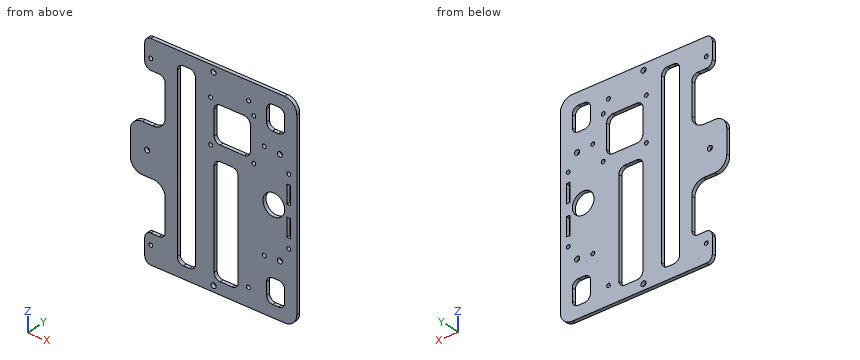
```python
from build123d import *

# Parameters (mm, degrees)
SKETCH1_W           = 138
SKETCH1_H           = 170
BOSS_EXTRUDE1_DEPTH = 3
SKETCH2_R           = 2.1
SKETCH2_W           = 29
SKETCH2_H           = 30
CUT_EXTRUDE1_DEPTH  = 3
SKETCH3_R           = 2.1
CUT_EXTRUDE2_DEPTH  = 219.981734398
SKETCH5_W           = 29
SKETCH5_H           = 35
CUT_EXTRUDE3_DEPTH  = 219.981734398
SKETCH6_R           = 1.6
SKETCH6_W           = 3.2
SKETCH6_H           = 15.2
CUT_EXTRUDE4_DEPTH  = 219.981734398
SKETCH9_W           = 29
SKETCH9_H           = 30
BOSS_EXTRUDE2_DEPTH = 3
SKETCH10_R          = 1.6
CUT_EXTRUDE5_DEPTH  = 219.981734398
FILLET1_R           = 10
FILLET2_R           = 10
SKETCH12_W          = 15
SKETCH12_H          = 150
CUT_EXTRUDE6_DEPTH  = 219.981734398
FILLET3_R           = 5
SKETCH13_R          = 9
SKETCH13_W          = 15
SKETCH13_H          = 20
CUT_EXTRUDE7_DEPTH  = 219.981734398
FILLET4_R           = 5
SKETCH14_W          = 27
SKETCH14_H          = 24
SKETCH14_R          = 1.6
BOSS_EXTRUDE3_DEPTH = 3
SKETCH15_R          = 1.6
CUT_EXTRUDE8_DEPTH  = 219.981734398
FILLET5_R           = 5
SKETCH16_W          = 20
SKETCH16_H          = 90
CUT_EXTRUDE9_DEPTH  = 219.981734398
FILLET6_R           = 5


with BuildPart() as part:
    # Sketch1 → Boss-Extrude1 (new body)
    with BuildSketch(Plane(origin=(0, 0, 0), x_dir=(1, 0, 0), z_dir=(0, 1, 0))):
        with Locations((69, 85)):
            Rectangle(SKETCH1_W, SKETCH1_H)
    extrude(amount=BOSS_EXTRUDE1_DEPTH)

    # Sketch2 → Cut-Extrude1 (cut)
    with BuildSketch(Plane(origin=(0, 3, 0), x_dir=(1, 0, 0), z_dir=(0, 1, 0))):
        with Locations(Location((69, 165, 0), (0, 0, 270))):
            Circle(SKETCH2_R)
        with Locations(Location((69, 5, 0), (0, 0, 270))):
            Circle(SKETCH2_R)
        with Locations((14.5, 155)):
            Rectangle(SKETCH2_W, SKETCH2_H)
        with Locations((123.5, 155)):
            Rectangle(SKETCH2_W, SKETCH2_H)
        with Locations((123.5, 15)):
            Rectangle(SKETCH2_W, SKETCH2_H)
        with Locations((14.5, 15)):
            Rectangle(SKETCH2_W, SKETCH2_H)
    extrude(amount=-CUT_EXTRUDE1_DEPTH, mode=Mode.SUBTRACT)

    # Sketch3 → Cut-Extrude2 (cut, through all)
    with BuildSketch(Plane(origin=(0, 3, 0), x_dir=(1, 0, 0), z_dir=(0, 1, 0))):
        with Locations(Location((14, 125, 0), (0, 0, 270))):
            Circle(SKETCH3_R)
        with Locations(Location((14, 45, 0), (0, 0, 270))):
            Circle(SKETCH3_R)
        with Locations(Location((14, 85, 0), (0, 0, 270))):
            Circle(SKETCH3_R)
        with Locations(Location((124, 45, 0), (0, 0, 90))):
            Circle(SKETCH3_R)
        with Locations(Location((124, 125, 0), (0, 0, 90))):
            Circle(SKETCH3_R)
    extrude(amount=-CUT_EXTRUDE2_DEPTH, mode=Mode.SUBTRACT)

    # Sketch5 → Cut-Extrude3 (cut, through all)
    with BuildSketch(Plane(origin=(0, 3, 0), x_dir=(1, 0, 0), z_dir=(0, 1, 0))):
        with Locations((14.5, 122.5)):
            Rectangle(SKETCH5_W, SKETCH5_H)
        with Locations((14.5, 47.5)):
            Rectangle(SKETCH5_W, SKETCH5_H)
    extrude(amount=-CUT_EXTRUDE3_DEPTH, mode=Mode.SUBTRACT)

    # Sketch6 → Cut-Extrude4 (cut, through all)
    with BuildSketch(Plane(origin=(0, 3, 0), x_dir=(1, 0, 0), z_dir=(0, 1, 0))):
        with Locations(Location((131.4, 113, 0), (0, 0, 270))):
            Circle(SKETCH6_R)
        with Locations(Location((131.4, 57, 0), (0, 0, 270))):
            Circle(SKETCH6_R)
        with Locations((131.4, 97.4)):
            Rectangle(SKETCH6_W, SKETCH6_H)
        with Locations((131.4, 72.6)):
            Rectangle(SKETCH6_W, SKETCH6_H)
    extrude(amount=-CUT_EXTRUDE4_DEPTH, mode=Mode.SUBTRACT)

    # Sketch9 → Boss-Extrude2 (add)
    with BuildSketch(Plane(origin=(0, 3, 0), x_dir=(1, 0, 0), z_dir=(0, 1, 0))):
        with Locations((123.5, 155)):
            Rectangle(SKETCH9_W, SKETCH9_H)
        with Locations((123.5, 15)):
            Rectangle(SKETCH9_W, SKETCH9_H)
    extrude(amount=-BOSS_EXTRUDE2_DEPTH)

    # Sketch10 → Cut-Extrude5 (cut, through all)
    with BuildSketch(Plane(origin=(0, 3, 0), x_dir=(1, 0, 0), z_dir=(0, 1, 0))):
        with Locations(Location((66.6, 60.4, 0), (0, 0, 270))):
            Circle(SKETCH10_R)
        with Locations(Location((102.4, 60.4, 0), (0, 0, 270))):
            Circle(SKETCH10_R)
        with Locations(Location((66.6, 24.6, 0), (0, 0, 270))):
            Circle(SKETCH10_R)
        with Locations(Location((102.4, 24.6, 0), (0, 0, 270))):
            Circle(SKETCH10_R)
        with BuildLine():
            Line((74.5, 57.5), (94.5, 57.5))
            ThreePointArc((94.5, 57.5), (98.035533906, 56.035533906), (99.5, 52.5))
            Line((99.5, 52.5), (99.5, 32.5))
            ThreePointArc((99.5, 32.5), (98.035533906, 28.964466094), (94.5, 27.5))
            Line((94.5, 27.5), (74.5, 27.5))
            ThreePointArc((74.5, 27.5), (70.964466094, 28.964466094), (69.5, 32.5))
            Line((69.5, 32.5), (69.5, 52.5))
            ThreePointArc((69.5, 52.5), (70.964466094, 56.035533906), (74.5, 57.5))
        make_face()
    extrude(amount=-CUT_EXTRUDE5_DEPTH, mode=Mode.SUBTRACT)

    # Fillet1
    fillet1_edges = [part.edges().sort_by_distance(p)[0] for p in [
        (0, 1.5, -105),
        (0, 1.5, -65),
        (138, 1.5, -170),
        (138, 1.5, 0),
        (29, 1.5, 0),
        (29, 1.5, -170),
    ]]
    fillet(fillet1_edges, radius=FILLET1_R)

    # Fillet2
    fillet2_edges = [part.edges().sort_by_distance(p)[0] for p in [
        (29, 1.5, -105),
        (29, 1.5, -65),
    ]]
    fillet(fillet2_edges, radius=FILLET2_R)

    # Sketch12 → Cut-Extrude6 (cut, through all)
    with BuildSketch(Plane(origin=(0, 3, 0), x_dir=(1, 0, 0), z_dir=(0, 1, 0))):
        with Locations((46.5, 85)):
            Rectangle(SKETCH12_W, SKETCH12_H)
    extrude(amount=-CUT_EXTRUDE6_DEPTH, mode=Mode.SUBTRACT)

    # Fillet3
    fillet3_edges = [part.edges().sort_by_distance(p)[0] for p in [
        (39, 1.5, -10),
        (39, 1.5, -160),
        (54, 1.5, -160),
        (54, 1.5, -10),
    ]]
    fillet(fillet3_edges, radius=FILLET3_R)

    # Sketch13 → Cut-Extrude7 (cut, through all)
    with BuildSketch(Plane(origin=(0, 3, 0), x_dir=(1, 0, 0), z_dir=(0, 1, 0))):
        with Locations(Location((119, 85, 0), (0, 0, 270))):
            Circle(SKETCH13_R)
        with Locations((120.5, 150)):
            Rectangle(SKETCH13_W, SKETCH13_H)
        with Locations((120.5, 20)):
            Rectangle(SKETCH13_W, SKETCH13_H)
    extrude(amount=-CUT_EXTRUDE7_DEPTH, mode=Mode.SUBTRACT)

    # Fillet4
    fillet4_edges = [part.edges().sort_by_distance(p)[0] for p in [
        (113, 1.5, -140),
        (113, 1.5, -160),
        (128, 1.5, -160),
        (128, 1.5, -140),
        (113, 1.5, -10),
        (113, 1.5, -30),
        (128, 1.5, -30),
        (128, 1.5, -10),
    ]]
    fillet(fillet4_edges, radius=FILLET4_R)

    # Sketch14 → Boss-Extrude3 (add)
    # profile 1 of 2: a face of its own
    with BuildSketch(Plane(origin=(0, 3, 0), x_dir=(1, 0, 0), z_dir=(0, 1, 0))):
        with Locations((25.5, 158)):
            Rectangle(SKETCH14_W, SKETCH14_H)
        with Locations(Location((17, 155, 0), (0, 0, 270))):
            Circle(SKETCH14_R, mode=Mode.SUBTRACT)
    # profile 2 of 2: a face of its own
    with BuildSketch(Plane(origin=(0, 3, 0), x_dir=(1, 0, 0), z_dir=(0, 1, 0))):
        with Locations((25.5, 12)):
            Rectangle(SKETCH14_W, SKETCH14_H)
        with Locations(Location((17, 15, 0), (0, 0, 270))):
            Circle(SKETCH14_R, mode=Mode.SUBTRACT)
    extrude(amount=-BOSS_EXTRUDE3_DEPTH)

    # Sketch15 → Cut-Extrude8 (cut, through all)
    with BuildSketch(Plane(origin=(0, 3, 0), x_dir=(1, 0, 0), z_dir=(0, 1, 0))):
        with Locations(Location((111, 44, 0), (0, 0, 270))):
            Circle(SKETCH15_R)
        with Locations(Location((111, 126, 0), (0, 0, 270))):
            Circle(SKETCH15_R)
        with Locations(Location((98, 155, 0), (0, 0, 270))):
            Circle(SKETCH15_R)
        with Locations(Location((98, 15, 0), (0, 0, 270))):
            Circle(SKETCH15_R)
    extrude(amount=-CUT_EXTRUDE8_DEPTH, mode=Mode.SUBTRACT)

    # Fillet5
    fillet5_edges = [part.edges().sort_by_distance(p)[0] for p in [
        (29, 1.5, -146),
        (12, 1.5, -146),
        (12, 1.5, -170),
        (12, 1.5, -24),
        (12, 1.5, 0),
        (29, 1.5, -24),
    ]]
    fillet(fillet5_edges, radius=FILLET5_R)

    # Sketch16 → Cut-Extrude9 (cut, through all)
    with BuildSketch(Plane(origin=(0, 3, 0), x_dir=(1, 0, 0), z_dir=(0, 1, 0))):
        with Locations((79.5, 115)):
            Rectangle(SKETCH16_W, SKETCH16_H)
    extrude(amount=-CUT_EXTRUDE9_DEPTH, mode=Mode.SUBTRACT)

    # Fillet6
    fillet6_edges = [part.edges().sort_by_distance(p)[0] for p in [
        (69.5, 1.5, -70),
        (69.5, 1.5, -160),
        (89.5, 1.5, -160),
        (89.5, 1.5, -70),
    ]]
    fillet(fillet6_edges, radius=FILLET6_R)


solid = part.part
```
Work out the finished part from the listing and answer in its coordinate system (mm). Give positions to 0.01 mm unless a question says otherwise; leave off trailing zeros. Loops run counter-clockwise (first coordinate to the right, second up) from the corner with the lowest first, then second, coordinate; pieces in that order, holes last. Notation, with made-up numbers: M 19.25,-1 L 56.25,-1 A11 ccw 56.25,9 Z; hole C -25.5,23.25 d3. An arc over 180 degrees is marked long. One line per item, written item: value. Start each with the question number.
1. Find section C-C (y = 1.05). State how many separate pieces and enclosed holes the cut face has, and give its area (3 significant figures).
2. Find the intervals of material crossed by probe 1 along X at (y, z) = (2.25, -34); probe 2 along Z at (x, y) = (66.6, 0.7); probe 3 along X at (y, z) = (1.5, -116), in increasing order.
3. Each of these flat-tipped pins is pushed along its axis until it touches: P1, Ø2.5, axis at x = 111, z = -126, coming from the +Y side; P2, Ø0.9, axis at y = 1, z = -159.5, coming from the -X side. Where does it stop, or does it pass through?
4. Find section B-B (z = -78). Give the vertices of the cut face in (x, y).
5. Find section A-A (z = -101). Give the vertices of the cut face in (x, y).
Reported:
1. separate pieces: 1
1. enclosed holes: 25
1. area: 14,500 mm²
2. probe 1: x = 29 to 39, 54 to 69.5, 99.5 to 138
2. probe 2: z = -170 to -62, -58.8 to -26.2, -23 to 0
2. probe 3: x = 29 to 39, 54 to 69.5, 89.5 to 138
3. P1: passes through
3. P2: stops at x = 12
4. outline: M 0,0 L 39,0 L 39,3 L 0,3 Z; M 54,0 L 69.5,0 L 69.5,3 L 54,3 Z; M 89.5,0 L 113.34,0 L 113.34,3 L 89.5,3 Z; M 124.66,0 L 129.8,0 L 129.8,3 L 124.66,3 Z; M 133,0 L 138,0 L 138,3 L 133,3 Z
5. outline: M 2,0 L 39,0 L 39,3 L 2,3 Z; M 54,0 L 69.5,0 L 69.5,3 L 54,3 Z; M 89.5,0 L 129.8,0 L 129.8,3 L 89.5,3 Z; M 133,0 L 138,0 L 138,3 L 133,3 Z
